Geometry check sheet. Reference: the model listing, model coordinates, mm. A direction names the side the tool comes from. Give positions to 0.01 mm unless a question says otherwise; leave off trailing zeros. Order: outer loops, then holes, each group sorted by start corner. A loop starts at its lowest first (then second) coordinate and runs counter-clockwise, first axis right, second up. Notation, with made-up numbers: M -12.75,18 L 28.25,18 A8 ccw 28.25,29 Z; hole C 19,-27.75 d2. An arc over 180 degrees is marked long. Answer as a JSON object with one key per item and string values. Group by question number.
Autodesk Inventor part; units mm, degrees
ref_plane "YZ Plane" through (0, 0, 0) normal (1, 0, 0) x (0, 1, 0)
ref_plane "XZ Plane" through (0, 0, 0) normal (0, 1, 0) x (-1, 0, 0)
sketch "Sketch1" plane through (0, 0, 0) normal (0, 1, 0) x (-1, 0, 0)
  circle A0 centre (0, 0) radius 20.75
  dimension "d0" = 41.5
extrude "Extrusion1" add sketch "Sketch1" along normal blind 30
sketch "Sketch4" plane through (0, 30, 0) normal (0, 1, 0) x (1, 0, 0)
  circle A0 centre (0, 0) radius 3.25
  dimension "d8" = 6.5
extrude "Extrusion4" cut sketch "Sketch4" against normal blind 15
sketch "Sketch5" plane through (0, 30, 0) normal (0, 1, 0) x (1, 0, 0)
  circle A0 centre (0, 0) radius 15.2932
extrude "Extrusion5" cut sketch "Sketch5" against normal blind 5
ref_plane "Work Plane1" through (0, 0, 10) normal (0, 0, 1) x (1, 0, 0)
sketch "Sketch6" plane through (0, 0, 10) normal (0, 0, 1) x (1, 0, 0)
  circle A0 centre (0, 20.8731) radius 1.5
  point P0 (0, 0)
  dimension "d14" = 3
extrude "Extrusion6" cut sketch "Sketch6" along normal mid plane 25
ref_plane "Work Plane2" through (0, 0, 20) normal (0, 0, 1) x (1, 0, 0)
sketch "Sketch7" plane through (0, 0, 20) normal (0, 0, 1) x (1, 0, 0)
  circle A0 centre (0, 20.8731) radius 2.3877
  point P0 (0, 0)
  point P1 (1.5, 20.8731)
extrude "Extrusion7" cut sketch "Sketch7" along normal mid plane 25
properties part number "ban"
1. Depth check by flat-ended pin: pin 1 (12 mm diameter, centred on x = -6, y = 19.5, fed in from -Z); pin 2 (8 mm diameter, centred on y = 25.5, z = 12, fed in from -X); pin 3 (3 mm diameter, centred on x = 1, z = 1, fed in from +Y). Enter the tip coordinate at first touch or a pass-through.
2. Thickness scan on line 1 along Y through (x, z) = (0, 6); line 2 along Z through (x, y) = (0, 19); line 3 along Z through (x, y) = (0, 26). Record the ranges inside material, lowest first. Write a range as [from, to].
3. Cross-section at D-D (y = 17). Record the cut outline in (x, z), and give its area (3 significant figures).
4. Cross-section at A-A (x = 0). Record the cut outline in (y, z), and give its area (3 significant figures).
5. Release check for a two-part mould opening along Y. For faces 1 (the flat face through (0, 15, 0)), 2 (the cylindrical face through (-0.2, 22.36, 5.22)), 3 (the cylindrical face through (-3.32, 27.54, 14.93)) record: released by +Y, released by -Y, zero draft, split by the parting line, or undercut.
6. Cross-section at B-B (z = 4.5). Record the cut outline in (x, y).
7. Access from +Z, -Z, +X, -X, +Y, -Y to the whole of each face (thin tool, end or side, straight path). Record for faces 4 (the cylindrical face through (-0.311, 18.506, 14.032)), 5 (the cylindrical face through (-19.8, 14.8, -6.2)), 6 (the flat face through (0, 25, -4)).
8. Cross-section at C-C (z = 0). Record the cut outline in (x, y), and give its area (3 significant figures).
Report:
{
 "1": {"pin 1": "stops at z = -20.75", "pin 2": "stops at x = -19.15", "pin 3": "stops at y = 15"},
 "2": {"line 1": "y = [0, 19.37], [22.37, 25]", "line 2": "z = [-20.75, -3.25], [3.25, 7.5]", "line 3": "z = [-20.75, -15.29], [15.29, 20.75]"},
 "3": {"outline": "C 0,0 d41.5; hole C 0,0 d6.5", "area": "1,320 mm2"},
 "4": {"outline": "M 0,-20.75 L 30,-20.75 L 30,-15.29 L 25,-15.29 L 25,-3.25 L 15,-3.25 L 15,3.25 L 19.37,3.25 L 19.37,7.5 L 18.49,7.5 L 18.49,20.75 L 0,20.75 Z; M 22.37,3.25 L 25,3.25 L 25,15.29 L 30,15.29 L 30,20.75 L 23.26,20.75 L 23.26,7.5 L 22.37,7.5 Z", "area": "951 mm2"},
 "5": {"face 1": "released by +Y", "face 2": "undercut", "face 3": "zero draft"},
 "6": {"outline": "M -20.26,0 L 20.26,0 L 20.26,30 L 14.62,30 L 14.62,25 L -14.62,25 L -14.62,30 L -20.26,30 Z; hole C 0,20.87 d3"},
 "7": {"face 4": "+Z", "face 5": "+Y, -Y", "face 6": "+Y"},
 "8": {"outline": "M -20.75,0 L 20.75,0 L 20.75,30 L 15.29,30 L 15.29,25 L 3.25,25 L 3.25,15 L -3.25,15 L -3.25,25 L -15.29,25 L -15.29,30 L -20.75,30 Z", "area": "1,030 mm2"}
}
